from build123d import *

# Parameters (mm, degrees)
EXTRUDE1_DEPTH     = 48.26
SKETCH3_OUTSIDE_W  = 133.914
SKETCH3_OUTSIDE_H  = 80.574
CUT_EXTRUDE1_DEPTH = 127
FILLET1_R          = 12.7
FILLET2_R          = 12.7


with BuildPart() as part:
    # Sketch1 → Extrude1 (new body)
    with BuildSketch(Plane(origin=(0, 0, 0), x_dir=(1, 0, 0), z_dir=(0, 1, 0))):
        Polygon((-44.45, 101.6), (44.45, 101.6), (44.45, 57.94375), (57.15, 50.8), (28.575, 0), (-28.575, 0), (-44.45, 50.8), align=None)
    extrude(amount=EXTRUDE1_DEPTH)

    # Sketch3 outside → Cut-Extrude1 (cut, symmetric)
    with BuildSketch(Plane.ZY.offset(44.45)):
        with Locations((-50.8, 24.13)):
            Rectangle(SKETCH3_OUTSIDE_W, SKETCH3_OUTSIDE_H)
        Polygon((0, 41.445288221), (-101.6, 48.26), (-101.6, 22.86), (-68.397585835, 20.632983436), (-57.94375, 9.084619968), (-25.4, 0), (0, 5.240594668), align=None, mode=Mode.SUBTRACT)
    extrude(amount=CUT_EXTRUDE1_DEPTH, both=True, mode=Mode.SUBTRACT)

    # Fillet1
    fillet1_edges = [part.edges().sort_by_distance(p)[0] for p in [
        (-44.45, 35.56, -101.6),
        (44.45, 35.56, -101.6),
        (0, 48.26, -101.6),
        (-44.45, 46.556322055, -76.2),
        (-36.5125, 43.148966165, -25.4),
        (42.8625, 43.148966165, -25.4),
        (50.8, 45.092223821, -54.371875),
        (44.45, 46.795901766, -79.771875),
    ]]
    fillet(fillet1_edges, radius=FILLET1_R)

    # Fillet2
    fillet2_edges = [part.edges().sort_by_distance(p)[0] for p in [
        (-40.48125, 3.545217548, -38.1),
        (-32.54375, 2.620297334, -12.7),
        (50.00625, 3.545217548, -38.1),
        (35.71875, 2.620297334, -12.7),
    ]]
    fillet(fillet2_edges, radius=FILLET2_R)


solid = part.part
Could you check a few things on this model? Use its own coordinates, in mm. A direction names the side the tool comes from. Round coordinates to 2 decimals unless told otherwise and drop trailing zeros. Order: outer loops, then holes, each group sorted by start corner. A loop starts at its lowest first (then second) coordinate and runs counter-clockwise, first axis right, second up.
(1) Please list where these lines run through material, in increasing order: line 1 along X through (y, z) = (26.5, -89); line 2 along Y through (x, z) = (10.5, -88.5); line 3 along X through (y, z) = (24, -42).
Response values:
line 1: x = -44.45 to 44.45
line 2: y = 21.98 to 47.37
line 3: x = -41.7 to 52.2
(2) Imagine slicing it at A-A (y = 25.5). Write out the boundary of the cut face in (x, z) (3 decimals).
Response values:
outline: (-44.45, -88.9) arc R12.7 ccw to (-31.75, -101.6) - (31.75, -101.6) arc R12.7 ccw to (44.45, -88.9) - (44.45, -57.944) - (57.15, -50.8) - (28.575, 0) - (-28.575, 0) - (-44.45, -50.8) - close
(3) Which directions (+Z, -Z, +X, -X, +Y, -Y) give clear straight access to the entire face, cutting with the end or side of a thin tool? Please do faces 1 (the cylindrical face through (-40.63, 42.48, -69.51)), 2 (the flat face through (44.45, 27, -74)), 3 (the cylindrical face through (40.83, 42.52, -73.11)).
Response values:
face 1: +Z, -X, +Y
face 2: -Z, +X, +Y, -Y
face 3: +X, +Y
(4) Imagine slicing it at B-B (x = -0.5). Write out the boundary of the cut face in (y, z).
Response values:
outline: (0, -25.4) - (9.08, -57.94) - (20.63, -68.4) - (22.86, -101.6) - (34.68, -101.6) arc R12.7 ccw to (47.35, -88.05) - (41.45, 0) - (5.24, 0) - close
(5) I'm going to push flat-ended pins straight in: pin 1 (4 mm diameter, centred on x = 37, y = 38, fed in from +Z); pin 2 (4 mm diameter, centred on x = -16, y = 17.5, fed in from -Z); pin 3 (10 mm diameter, centred on y = 9, z = -12.5, fed in from -X). Where does each tip first touch, or does it pass through?
Response values:
pin 1: stops at z = -15.96
pin 2: stops at z = -67.37
pin 3: stops at x = -33.59
